Geometry: final body of the model. Coordinates: model frame, mm. Face numbers are marked on the shaded views. A direction names the side the tool comes from. Give positions to 0.01 mm unless a question says otherwise; leave off trailing zeros. Write each loop counter-clockwise with the first axis right and the second up, starting at its lowest first coordinate (ties: lowest second). Pieces come first, ordered by that corner, then holes. Notation, with made-up numbers: (-29, 56) -> (-3, 56) arc R18 cw to (-3, 66) -> close; hole circle Ø5 at (-26, -33). An arc over 180 degrees is marked (long way). Answer in a Markdown table with one row per item. Add a question column.
Item 1: Draft query along Z for the marked faces 4, 5 and 6. Return one class per face: +Z half, -Z half, draft (parallel to the pull), parting line (faces both ways), or undercut.
Item 2: Material intervals for probe 1 along Z at (x, y) = (0.05, 0); probe 2 along Z at (x, y) = (-0.3, 0); probe 3 along Y at (x, z) = (17.5, -1), sorted ascending. Write a range as from..to.
Item 3: Access query for the marked faces 1, 2 and 3. Directions: +Z, -Z, +X, -X, +Y, -Y. A direction counts if a zero-diameter tool reaches every point of the face in a straight line with its end or side. Return the directions, or none.
Item 4: First-contact query: P1, Ø2, axis at x = 10, y = -2, coming from the -Z side; P2, Ø1.5, axis at x = 14, y = -1.5, coming from the -Z side; P3, Ø1.5, axis at x = 11, z = -1, coming from the +Y side. Flat tips, straight axial feed; report the tip coordinate or a pass-through.
Item 5: Section query A-A on x = 8. Output: boundary loops of the cut face in (y, z).
Autodesk Inventor part; units mm, degrees
ref_plane "Work Plane1" through (12.5, 0, 0) normal (0, 0.5, 0.866) x (1, 0, 0)
ref_plane "YZ Plane" through (0, 0, 0) normal (1, 0, 0) x (0, 1, 0)
ref_plane "XZ Plane" through (0, 0, 0) normal (0, 1, 0) x (-1, 0, 0)
sketch "Sketch1" plane through (0, 0, 0) normal (0, 0, 1) x (1, 0, 0)
  line L0 (1.0774, 0) -> (25, 0)
  line L1 (25, 0) -> (25, 2)
  line L2 (25, 2) -> (0, 2)
  line L3 (0, 2) -> (0, 3.5)
  line L4 (0, 3.5) -> (-2.8, 3.5)
  line L5 (-2.8, 3.5) -> (-2.8, 1.7321)
  line L6 (-2.8, 1.7321) -> (-1.2, 1.7321)
  line L7 (-1.2, 1.7321) -> (-0.7774, 1)
  line L8 (-8.36, 0) -> (30.56, 0)
  line L9 (0, -0.7) -> (0, 4.2)
  line L10 (-0.7774, 1) -> (0.5, 1)
  line L11 (0.5, 1) -> (1.0774, 0)
  line L12 (-2.8, 1.7321) -> (-2.8, 0) construction
  line L13 (-2.8, 3.1) -> (-2.4, 3.5)
  dimension "d0" = 2.8
  dimension "d1" = 1.6
  dimension "d2" = 60
  dimension "d3" = 4
  dimension "d4" = 3.4641
  dimension "d5" = 7
  dimension "d15" = 3.3
  dimension "d16" = 2
  dimension "d17" = 25
  dimension "d32" = 45
  dimension "d33" = 0.4
revolve "Body" add sketch "Sketch1" angle 360 about axis through (1.0774, 0, 0) along (1, 0, 0) contours L11 L10 L9 L2 L1 L0 | L10 L7 L6 L5 L13 L4 L3 L9 | L13 L5 L4
revolve "Chamfer2" cut sketch "Sketch1" angle 360 about axis through (-10, 0, 0) along (1, 0, 0) contours L13 L5 L4
sketch "Sketch2" plane through (-2.8, 0, 0) normal (-1, 0, 0) x (0, 0, 1)
  circle A0 centre (0, 0) radius 1.7321
  line L0 (0, -4.9) -> (0, 4.9)
  line L1 (-4.9, 0) -> (4.9, 0)
  line L2 (1.7321, 0) -> (0.866, -1.5)
  line L3 (0.866, -1.5) -> (-0.866, -1.5)
  line L4 (-0.866, -1.5) -> (-1.7321, 0)
  line L5 (-1.7321, 0) -> (-0.866, 1.5)
  line L6 (-0.866, 1.5) -> (0.866, 1.5)
  line L7 (0.866, 1.5) -> (1.7321, 0)
extrude "Slot" add sketch "Sketch2" against normal up to next contours L7 A0 | A0 L2 | L6 L0 A0 | A0 L0 L3 | L0 L6 A0 | A0 L3 L0 | L4 A0 | A0 L5
thread "Thread"
chamfer "Chamfer1" distance 0.4294 distance2 0.4294 1 edges at (25, -2, 0) measured on face at (25, 0.6473, 0.1595)
ref_plane "Work Plane1" through (12.5, 0, 0) normal (0, 0.5, 0.866) x (1, 0, 0)
equation "\"d0\" = KOH"
equation "\"d1\" = INTI"
equation "\"d3\" = GD"
equation "\"d4\" = 1.1547 * SW"
equation "\"d5\" = KOD"
equation "\"d15\" = INFT"
equation "\"d16\" = SDT"
equation "\"d17\" = NLG"
equation "\"d33\" = Cham"
equation "\"d7\" = GEL"
equation "\"d9\" = -0.5 * SPD + 0.5 * GD"
equation "\"d12\" = GUL"
equation "\"GD\" = NND"
equation "\"NLG\" = 25"
equation "\"GEL\" = 14"
equation "\"KOD\" = 7"
equation "\"KOH\" = 2.8"
equation "\"GUL\" = 0.61345 * PTC"
equation "\"SW\" = 3"
equation "\"INTI\" = 1.6"
equation "\"SPD\" = NND - 1.2269 * PTC"
equation "\"SDT\" = 2"
equation "\"INFT\" = 3.3"
equation "\"Cham\" = 0.4"
equation "\"TOA\" = 30deg"
equation "\"GD1\" = THREADDIA - 1.2269 * PTC"
equation "\"THREADDIA\" = 4"
equation "\"BDM\" = NND"
equation "\"FAWI\" = 45deg"
equation "\"RR\" = 0.1 * NND"
equation "\"PTC\" = 0.7"
equation "\"NND\" = 4"
equation "\"FAWI1\" = 45deg"
equation "\"GAL\" = 0.61345 * PTC"
equation "\"E0\" = 1.155 * SW"
properties part number "DIN 6912 - M4 x 25" material "Steel, Mild"
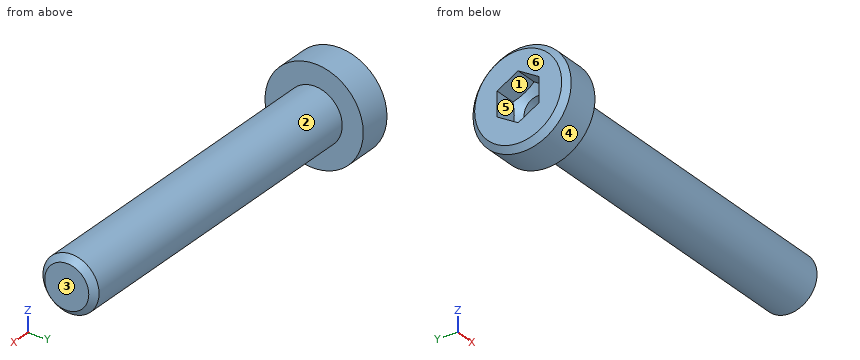
Findings below:
| question | item | result |
|---|---|---|
| 1 | face 4 | parting line |
| 1 | face 5 | undercut |
| 1 | face 6 | draft |
| 2 | probe 1 | z = -2..-1, 1..2 |
| 2 | probe 2 | z = -3.5..-1, 1..3.5 |
| 2 | probe 3 | y = -1.73..1.73 |
| 3 | face 1 | -X |
| 3 | face 2 | +X |
| 3 | face 3 | +Z, -Z, +X, +Y, -Y |
| 4 | P1 | stops at z = -1.73 |
| 4 | P2 | stops at z = -1.85 |
| 4 | P3 | stops at y = 1.98 |
| 5 | outline | circle Ø4 at (0, 0) |
